Geometry check sheet. Reference: the model listing, model coordinates, mm. A direction names the side the tool comes from. Coordinates: 2 decimals unless noted, no trailing zeros. Write each loop counter-clockwise with the first axis right and the second up, starting at its lowest first coordinate (ties: lowest second). Pieces come first, ordered by that corner, then holes. Notation, with made-up numbers: (83, 89.5) -> (133, 89.5) arc R35 cw to (133, 128.5) -> close; hole circle Ø11 at (72.25, -16.5). An arc over 180 degrees is marked (long way). Answer in a Markdown table with one row per item. Add a question column.
1. Set-up check for faces 3 (the flat face through (-39.88, 25.74, 47.47)), 4 (the flat face through (25.2, -51.7, 47.5)), 5 (the flat face through (-1, 1, 5)): record each of +Z, -Z, +X, -X, +Y, -Y from which the full face is reachable in a straight line by a thin tool's end or side.
2. Cross-section at A-A on x = 0. Give the number of separate pieces and of enclosed holes in the cut face, and give its area (3 significant figures).
3. Mould release check, pull along Y, two halves, no side actions. Record for faces 1 (the flat face through (0, 47, 9.828)), 2 (the flat face through (39.88, -25.74, 47.47)): pulls with the +Y half, pulls with the -Y half, needs draft (parallel to the pull), parting line crosses it, or undercut.
4. Cross-section at B-B on y = 0. Record the cut outline in (x, z).
5. Depth check by flat-ended pin: P1, Ø1.5, axis at y = 56, z = 60, coming from the +X side; P2, Ø6, axis at y = 43.5, z = 70.5, coming from the -X side; P3, Ø19.5, axis at x = -36.5, y = -36.5, coming from the -Z side; P4, Ø5, axis at y = -22.5, z = 23, coming from the -X side. Enter the tip coordinate at first touch or a pass-through.
6. Scan lines: L1, parallel to X at y = 55, z = 41.5; L2, parallel to Y at x = -40.5, z = 84; L3, parallel to Z at x = 4, y = 47. Record each from-to range of solid material in increasing order. Write a range as from..to.
```python
from build123d import *

# Parameters (mm, degrees)
F2_W            = 20
F2_H            = 76.3443418741
F3_REACH        = 138.9215837294
F3_COPIES_COUNT = 8
F5_W            = 20
F5_H            = 76.3443418741
F6_REACH        = 213.9215837294
F6_COPIES_COUNT = 10


# Not quite as in the source:
# - a pattern or mirror of a feature is missing from the dataset's text; its kind, count and spacing are read off the source's solid


with BuildPart() as f1:
    # F0 (on Front) → F1 (revolve)
    with BuildSketch(Plane.XZ):
        with BuildLine():
            Line((0, 5), (0, 0))
            Line((0, 0), (60, 0))
            Line((60, 0), (60, 96))
            Line((60, 96), (55, 96))
            Line((55, 96), (55, 5))
            Line((55, 5), (50, 5))
            Line((50, 5), (50, 96))
            Line((50, 96), (45, 96))
            Line((45, 96), (45, 10))
            ThreePointArc((45, 10), (43.5355339059, 6.4644660941), (40, 5))
            Line((40, 5), (0, 5))
        make_face()
    revolve(axis=Axis((0, 0, 2.5), (0, 0, 1)))

    f3_end = f1.faces().sort_by_distance((-50, 0, 50.5))[0]
    # F2 (on Front) → F3 (cut, up to a face of the model that its end follows)
    with BuildSketch(Plane.XZ):
        with Locations((0, 48)):
            Rectangle(F2_W, F2_H)
    f3_long = extrude(amount=F3_REACH, mode=Mode.PRIVATE)
    f3 = split(f3_long, bisect_by=f3_end, keep=Keep.BOTTOM, mode=Mode.PRIVATE)
    add(f3, mode=Mode.SUBTRACT)

    # F3_copies: F3 ×8 about axis
    f3_copies_axis = Axis((0, 0, 0), (0, 0, 1))
    for i in range(1, F3_COPIES_COUNT):
        add(f3.rotate(f3_copies_axis, i * 360 / F3_COPIES_COUNT), mode=Mode.SUBTRACT)

    f6_end = f1.faces().sort_by_distance((-55, 0, 50.5))[0]
    # F5 (on offset) → F6 (cut, up to a face of the model that its end follows)
    with BuildSketch(Plane.XZ.offset(75)):
        with Locations((0, 48)):
            Rectangle(F5_W, F5_H)
    f6_long = extrude(amount=-F6_REACH, mode=Mode.PRIVATE)
    f6 = split(f6_long, bisect_by=f6_end, keep=Keep.ALL, mode=Mode.PRIVATE).solids().sort_by_distance((0, -75, 48))[0]
    add(f6, mode=Mode.SUBTRACT)

    # F6_copies: F6 ×10 about axis
    f6_copies_axis = Axis((0, 0, 0), (0, 0, 1))
    for i in range(1, F6_COPIES_COUNT):
        add(f6.rotate(f6_copies_axis, i * 360 / F6_COPIES_COUNT), mode=Mode.SUBTRACT)


solid = f1.part
```
Results found:
| question | item | result |
|---|---|---|
| 1 | face 3 | none |
| 1 | face 4 | +X |
| 1 | face 5 | +Z |
| 2 | separate pieces | 5 |
| 2 | enclosed holes | 0 |
| 2 | area | 904 mm^2 |
| 3 | face 1 | needs draft |
| 3 | face 2 | undercut |
| 4 | outline | (-60, 0) -> (60, 0) -> (60, 96) -> (55, 96) -> (55, 5) -> (50, 5) -> (50, 9.83) -> (45, 9.83) arc R5 cw to (40, 5) -> (-40, 5) arc R5 cw to (-45, 9.83) -> (-50, 9.83) -> (-50, 5) -> (-55, 5) -> (-55, 96) -> (-60, 96) -> close; (-50, 86.17) -> (-45, 86.17) -> (-45, 96) -> (-50, 96) -> close; (45, 86.17) -> (50, 86.17) -> (50, 96) -> (45, 96) -> close |
| 5 | P1 | stops at x = 23.4 |
| 5 | P2 | stops at x = -44.27 |
| 5 | P3 | stops at z = 0 |
| 5 | P4 | stops at x = -45.83 |
| 6 | L1 | x = -23.98..-10, 10..23.98 |
| 6 | L2 | y = -38.73..-37.21, -26.36..-19.62, 19.62..26.36, 37.21..38.73 |
| 6 | L3 | z = 0..9.83, 86.17..96 |
